Part model, mm, in its own coordinate system. A direction names the side the tool comes from. Give positions to 0.01 mm unless a question says otherwise; leave off trailing zeros. Order: outer loops, then holes, each group sorted by start corner. A loop starts at its lowest first (then second) coordinate and runs counter-clockwise, first axis right, second up. Notation, with made-up numbers: M 26.5,17.25 L 81.5,17.25 A28 cw 81.5,50.25 Z; hole C 69.5,60 d4. An arc over 180 degrees is marked long. Return JSON: item names as keys, results as strings.
from build123d import *

# Parameters (mm, degrees)
SKIZZE1_R                       = 3
AUFSATZ_LINEAR_AUSTRAGEN1_DEPTH = 25
AUSTRAGUNG1_PITCH               = 22
AUSTRAGUNG1_HEIGHT              = 16.5
AUSTRAGUNG1_RADIUS              = 9
AUSTRAGUNG1_START_ANGLE         = 90
SKIZZE3_R                       = 3
SKIZZE4_R                       = 3
AUFSATZ_LINEAR_AUSTRAGEN2_DEPTH = 20
FASE1_SIZE                      = 1


with BuildPart() as part:
    # Skizze1 → Aufsatz-Linear austragen1 (new body)
    with BuildSketch(Plane.XY):
        Circle(SKIZZE1_R)
    extrude(amount=AUFSATZ_LINEAR_AUSTRAGEN1_DEPTH)

    # Austragung1: sweep along a helix
    with BuildLine() as austragung1_path:
        add(Helix(AUSTRAGUNG1_PITCH, AUSTRAGUNG1_HEIGHT, AUSTRAGUNG1_RADIUS, center=(-9, 0, 25), direction=(0, -1, 0), mode=Mode.PRIVATE).rotate(Axis((-9, 0, 25), (0, -1, 0)), AUSTRAGUNG1_START_ANGLE))
    # Skizze3 → Austragung1 (sweep)
    with BuildSketch(Plane.XY.offset(25)):
        Circle(SKIZZE3_R)
    sweep(path=austragung1_path.line, is_frenet=True)

    # Skizze4 → Aufsatz-Linear austragen2 (add)
    with BuildSketch(Plane(origin=(-9, 0, 0), x_dir=(0, 0, -1), z_dir=(1, 0, 0))):
        with Locations((-16, -16.5)):
            Circle(SKIZZE4_R)
    extrude(amount=AUFSATZ_LINEAR_AUSTRAGEN2_DEPTH)

    # Fase1
    fase1_edges = [part.edges().sort_by_distance(p)[0] for p in [
        (11, -16.5, 19),
        (-3, 0, 0),
    ]]
    chamfer(fase1_edges, length=FASE1_SIZE)


solid = part.part
Q1. Probe line 1 along Y through (x, z) = (0, 24.5); line 2 along X through (y, z) = (-0.75, 24.5); line 3 along Y through (x, z) = (8, 14). List the from-to ranges inside material, lowest first.
Established:
{"line 1": "y = -3 to 3", "line 2": "x = -2.9 to 2.9", "line 3": "y = -18.74 to -14.26"}
Q2. Band-saw the part on A-A (z = 4.5). Give the cut face in (x, y), then the cut area to 3 significant figures.
Established:
{"outline": "C 0,0 d6", "area": "28.3 mm²"}
Q3. Pin check, flat tips, straight feed: pin 1 (5 mm diameter, centred on y = -7, z = 5.5, fed in from +X); pin 2 (5 mm diameter, centred on y = -12.5, z = 23, fed in from +X); pin 3 (10 mm diameter, centred on x = -5.5, y = -9.5, fed in from +Z); pin 4 (6 mm diameter, centred on x = 1.5, z = 11.5, fed in from -Y). Stop position of each tip, or through.
Established:
{"pin 1": "passes through", "pin 2": "stops at x = -13.18", "pin 3": "stops at z = 36.99", "pin 4": "stops at y = -19.1"}
Q4. Two-plate mould, pull along Y, no slides. Class faces 3 (the flat face through (0, 0, 0)), 4 (the cylindrical face through (0.37, -19.43, 16.65)): +Y half, -Y half, draft (parallel to the pull), parting line (faces both ways), or undercut.
Established:
{"face 3": "draft", "face 4": "undercut"}
Q5. 3-axis set-ups, long thin cutter, end or side, ignore diameter. For faces 1 (the cylindrical face through (-3, 0, 13)), 2 (the flat face through (11, -16, 16)): which of +Z, -Z, +X, -X, +Y, -Y reach the whole face in a straight line?
Established:
{"face 1": "-Z", "face 2": "+Z, -Z, +X, +Y, -Y"}
